Autodesk Inventor part; units mm, degrees
ref_plane "YZ Plane" through (0, 0, 0) normal (1, 0, 0) x (0, 1, 0)
ref_plane "XZ Plane" through (0, 0, 0) normal (0, 1, 0) x (-1, 0, 0)
ref_plane "XY Plane" through (0, 0, 0) normal (0, 0, 1) x (1, 0, 0)
sketch "Sketch1" plane through (0, 0, 0) normal (0, 1, 0) x (-1, 0, 0)
  point P0 (0, 0)
sketch "Sketch2" plane through (0, 0, 0) normal (0, 1, 0) x (-1, 0, 0)
  circle A0 centre (0, 0) radius 4.5
  dimension "d0" = 9
extrude "Extrusion1" add sketch "Sketch2" along normal blind 5
sketch "Sketch3" plane through (0, 0, 0) normal (0, -1, 0) x (1, 0, 0)
  circle A0 centre (0, 0) radius 3.25
  dimension "d3" = 6.5
extrude "Extrusion2" cut sketch "Sketch3" against normal blind 3
sketch "Sketch4" plane through (0, 5, 0) normal (0, 1, 0) x (1, 0, 0)
  circle A0 centre (0, 0) radius 0.5
  dimension "d6" = 1
extrude "Extrusion3" cut sketch "Sketch4" along normal blind 3
sketch "Sketch5" plane through (0, 5, 0) normal (0, 1, 0) x (1, 0, 0)
  circle A0 centre (0, 0) radius 0.5
  dimension "d9" = 1
extrude "Extrusion4" cut sketch "Sketch5" along normal blind 3
sketch "Sketch6" plane through (0, 5, 0) normal (0, 1, 0) x (1, 0, 0)
  circle A0 centre (0, 0) radius 0.5
  dimension "d12" = 1
extrude "Extrusion5" cut sketch "Sketch6" against normal blind 3
properties part number "Explo base"
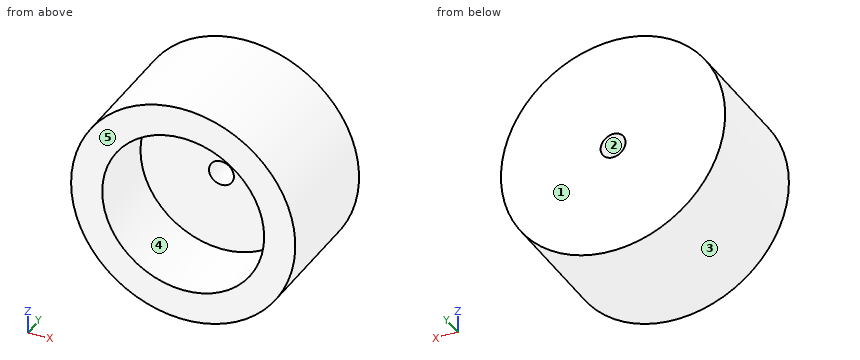
Work out the finished part from the listing and answer in its coordinate system (mm). Face numbers are marked on the shaded views. A direction names the side the tool comes from. Coordinates: 2 decimals unless noted, no trailing zeros. Loops run counter-clockwise (first coordinate to the right, second up) from the corner with the lowest first, then second, coordinate; pieces in that order, holes last. Notation, with made-up numbers: (72, 9.25) -> (100, 9.25) arc R16 cw to (100, 25.25) -> close; hole circle Ø4 at (-27, 42.5). An arc over 180 degrees is marked (long way). Write each question's results on one line, items separated by ' | '. Start each with the question number.
1) Find section B-B on y = 3.95. Determine the outline of the cut face in (x, z), then the cut area to 3 significant figures.
2) Find section C-C on z = -1. Determine the outline of the cut face in (x, y).
3) Find section A-A on x = 0. Determine the outline of the cut face in (y, z).
4) The mould has two halves that part along X. Classify the marked faces 1, 2 and 3: pulls with the +X half, pulls with the -X half, needs draft (parallel to the pull), parting line crosses it, or undercut.
5) For the marked faces 4 and 5, determine the directions among +Z, -Z, +X, -X, +Y, -Y from which every point of the face is accessible in a straight line to the end or side of a thin tool.
6) Flat-ended cylindrical pins translate along their axes: P1, Ø3, axis at y = 3, z = -3.5, coming from the -X side; P2, Ø1, axis at y = 2.5, z = 3, coming from the -X side. Find the tip coordinate at first contact, or state that the pin passes through.
7) Consider line 1 along Z through (x, y) = (0, 4.45); line 2 along Z through (x, y) = (0, 2.3); line 3 along Y through (x, z) = (-2, 1.75). Determine where each line is inside the solid, lowest interval first.
8) Find section D-D on x = -2. Determine the outline of the cut face in (y, z).
Response values:
1) outline: circle Ø9 at (0, 0); hole circle Ø1 at (0, 0) | area: 62.8 mm^2
2) outline: (-4.39, 0) -> (-3.09, 0) -> (-3.09, 3) -> (3.09, 3) -> (3.09, 0) -> (4.39, 0) -> (4.39, 5) -> (-4.39, 5) -> close
3) outline: (0, -4.5) -> (5, -4.5) -> (5, -0.5) -> (3, -0.5) -> (3, -3.25) -> (0, -3.25) -> close; (0, 3.25) -> (3, 3.25) -> (3, 0.5) -> (5, 0.5) -> (5, 4.5) -> (0, 4.5) -> close
4) face 1: needs draft | face 2: undercut | face 3: parting line crosses it
5) face 4: -Y | face 5: +Z, -Z, +X, -X, -Y
6) P1: stops at x = -4.03 | P2: stops at x = -3.74
7) line 1: z = -4.5 to -0.5, 0.5 to 4.5 | line 2: z = -4.5 to -3.25, 3.25 to 4.5 | line 3: y = 3 to 5
8) outline: (0, -4.03) -> (5, -4.03) -> (5, 4.03) -> (0, 4.03) -> (0, 2.56) -> (3, 2.56) -> (3, -2.56) -> (0, -2.56) -> close
